The listing builds one solid part. Answer for the finished solid, in the listing's coordinates (mm). A direction names the side the tool comes from. Give positions to 0.01 mm unless a question says otherwise; leave off trailing zeros. Write each loop counter-clockwise with the first axis right and the second up, starting at its lowest first coordinate (ties: lowest second). Pieces come first, ordered by that corner, then holes. Notation, with made-up numbers: M 80.5,81.5 L 135.5,81.5 A14 cw 135.5,97.5 Z; hole C -5.5,6 d6. An arc over 180 degrees is marked long. Answer as a JSON object with one key per item and string values.
```python
from build123d import *

# Parameters (mm, degrees)
DODANIE_WYCI_GNI_CIE1_DEPTH      = 6.5
DODANIE_WYCI_GNI_CIE1_DEPTH_BACK = 6
SZKIC1_R                         = 1.05
SZKIC2_R                         = 1.55
DODANIE_WYCI_GNI_CIE2_DEPTH      = 1
ZAOKR_GLENIE1_R                  = 1.55


with BuildPart() as part:
    # Szkic1 → Dodanie-wyciągnięcie1 (new, two sides: drawn at the far end of the back side and taken through both)
    with BuildSketch(Plane.XY.offset(-DODANIE_WYCI_GNI_CIE1_DEPTH_BACK)):
        Circle(SZKIC1_R)
    extrude(amount=DODANIE_WYCI_GNI_CIE1_DEPTH + DODANIE_WYCI_GNI_CIE1_DEPTH_BACK)

    # Szkic2 → Dodanie-wyciągnięcie2 (add)
    with BuildSketch(Plane.XY.offset(6.5)):
        Circle(SZKIC2_R)
    extrude(amount=DODANIE_WYCI_GNI_CIE2_DEPTH)

    # Zaokrąglenie1
    # the kernel refuses this fillet: 1.55 mm, written as the material it takes off along each edge
    with BuildSketch(Plane(origin=(0, 0, 7.5), x_dir=(1, 0, 0), z_dir=(0, -1, 0))) as zaokr_glenie1_piece_1:
        with BuildLine():
            CenterArc((0.100862325, -1.55), ZAOKR_GLENIE1_R, 20.783559596, 69.216440404)
            Line((0.100862325, 0), (0.100862325, 0.031))
            Line((0.100862325, 0.031), (1.55, 0.031))
            Line((1.55, 0.031), (1.581, 0))
            ThreePointArc((1.581, 0), (1.581, -0.5), (1.578982753, -0.989))
            Line((1.578982753, -0.989), (1.55, -1))
        make_face()
    revolve(axis=Axis((0, 0, 7.5), (0, 0, 1)), mode=Mode.SUBTRACT)


solid = part.part
```
1. For faces 1 (the flat face through (0, 0, -6)), 2 (the cylindrical face through (1, 0.32, 0.16)), determine the directions among +Z, -Z, +X, -X, +Y, -Y from which every point of the face is accessible in a straight line to the end or side of a thin tool.
Verdict:
{"face 1": "-Z, +X, -X, +Y, -Y", "face 2": "-Z"}
2. A cutting plane is placed at A-A, the plane z = -1.25. Give the vertices of the cut face in (x, y), plus the area to 3 significant figures.
Verdict:
{"outline": "C 0,0 d2.1", "area": "3.46 mm2"}
3. Consider line 1 along Y through (x, z) = (-0.8, -5.25); line 2 along X through (y, z) = (0.1, 3); line 3 along X through (y, z) = (-0.5, 4.5). Determine where each line is inside the solid, lowest interval first.
Verdict:
{"line 1": "y = -0.68 to 0.68", "line 2": "x = -1.05 to 1.05", "line 3": "x = -0.92 to 0.92"}
